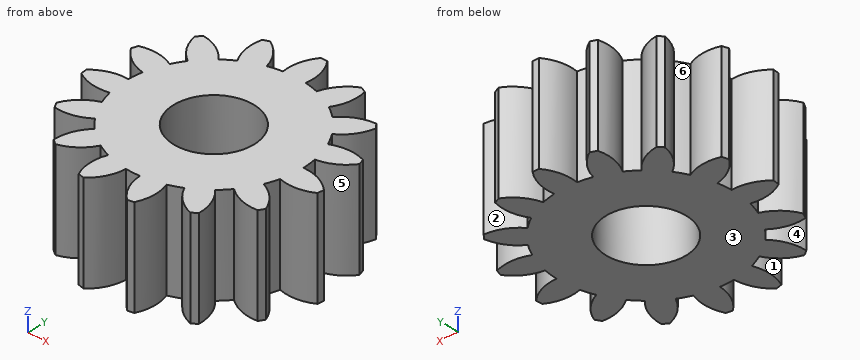
from build123d import *

# Parameters (mm, degrees)
ESBO_O1_R                = 9.374
RESSALTO_EXTRUS_O1_DEPTH = 10.4
RESSALTO_EXTRUS_O2_START = -10.4
RESSALTO_EXTRUS_O2_DEPTH = 10.4
PADR_OCIRCULAR1_COUNT    = 15
ESBO_O4_R                = 4.25
CORTE_EXTRUS_O1_DEPTH    = 10.4


with BuildPart() as part:
    # Esboço1 → Ressalto-extrusão1 (new body)
    with BuildSketch(Plane.XY):
        Circle(ESBO_O1_R)
    extrude(amount=RESSALTO_EXTRUS_O1_DEPTH)

    # Esboço2 → Ressalto-extrusão2 (add)
    with BuildSketch(Plane.XY.offset(10.4).offset(RESSALTO_EXTRUS_O2_START)):
        with BuildLine():
            Line((-0.337, 12.75), (0.337, 12.75))
            ThreePointArc((0.337, 12.75), (1.131844214, 11.112718069), (1.216843597, 9.294684915))
            ThreePointArc((1.216843597, 9.294684915), (0, 9.374), (-1.216843597, 9.294684915))
            ThreePointArc((-1.216843597, 9.294684915), (-1.131844214, 11.112718069), (-0.337, 12.75))
        make_face()
    ressalto_extrus_o2 = extrude(amount=RESSALTO_EXTRUS_O2_DEPTH)

    # PadrãoCircular1: Ressalto-extrusão2 ×15 about axis
    padr_ocircular1_axis = Axis((0, 0, 0), (0, 0, 1))
    for i in range(1, PADR_OCIRCULAR1_COUNT):
        add(ressalto_extrus_o2.rotate(padr_ocircular1_axis, i * 360 / PADR_OCIRCULAR1_COUNT))

    # Esboço4 → Corte-extrusão1 (cut)
    with BuildSketch(Plane.XY.offset(10.4)):
        Circle(ESBO_O4_R)
    extrude(amount=-CORTE_EXTRUS_O1_DEPTH, mode=Mode.SUBTRACT)


solid = part.part
Input: part model. Units: mm. Frame: model coordinates. Face numbers are marked on the shaded views. A direction names the side the tool comes from. Coordinates: 2 decimals unless noted, no trailing zeros. Loops run counter-clockwise (first coordinate to the right, second up) from the corner with the lowest first, then second, coordinate; pieces in that order, holes last.
(1) Set-up query: the marked faces 4, 5 and 6. Return all of +Z, -Z, +X, -X, +Y, -Y with unobstructed straight access to the full face (end or side cutting, diameter ignored); none if empty.
(2) Section A-A on x = 0. Return the cut outline in (y, z), then the cut area to 3 significant figures.
(3) First-contact query: pin 1 Ø3 at (y, z) = (9.5, 7) entering from +X; pin 2 Ø4 at (x, y) = (-0.5, 8.5) entering from -Z; pin 3 Ø2 at (y, z) = (-5.5, 8.5) entering from -X; pin 4 Ø5 at (x, y) = (0, 0) entering from +Z. Flat tips, straight axial feed; report the tip coordinate or a pass-through.
(4) Pull-direction query (Y, two-part tool) for the marked faces 1, 2 and 3; classes: released by +Y, released by -Y, zero draft, split by the parting line, or undercut.
(5) Material intervals for probe 1 along Y at (x, z) = (0, 2.5); probe 2 along Y at (x, z) = (-9.75, 2.75); probe 3 along X at (y, z) = (-9.25, 10), sorted ascending.
Data:
1. face 4: +Z, -Z, -X
1. face 5: +Z, -Z, +X
1. face 6: +Z, -Z
2. outline: (-9.37, 0) - (-4.25, 0) - (-4.25, 10.4) - (-9.37, 10.4) - close; (4.25, 0) - (12.75, 0) - (12.75, 10.4) - (4.25, 10.4) - close
2. area: 142 mm2
3. pin 1: stops at x = 9.7
3. pin 2: stops at z = 0
3. pin 3: stops at x = -11.21
3. pin 4: passes through
4. face 1: undercut
4. face 2: released by +Y
4. face 3: zero draft
5. probe 1: y = -9.37 to -4.25, 4.25 to 12.75
5. probe 2: y = -6.67 to -4.2, -2.3 to 0.24, 1.83 to 4.46
5. probe 3: x = -7.71 to -5.19, -3.26 to 3.26, 5.19 to 7.71
